The listing builds one solid part. Answer for the finished solid, in the listing's coordinates (mm). Coordinates: 2 decimals unless noted, no trailing zeros. Order: outer loops, then holes, each group sorted by start corner. A loop starts at its lowest first (then second) coordinate and runs counter-clockwise, first axis right, second up. Notation, with made-up numbers: (48, -15) -> (62, -15) arc R22 ccw to (62, 5) -> close; hole circle Ø6 at (39.5, -25). An arc over 180 degrees is marked (long way). Return JSON: item names as keys, results as strings.
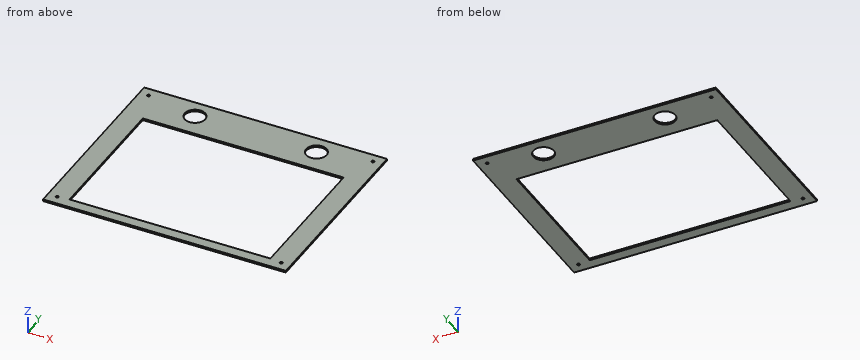
```python
from build123d import *

# Parameters (mm, degrees)
SKETCH_1_W          = 260
SKETCH_1_H          = 210
EXTRUDE_1_DEPTH     = 2
SKETCH_2_R          = 11
CUT_EXTRUDE_1_DEPTH = 2
SKETCH_3_R          = 1.5
CUT_EXTRUDE_2_DEPTH = 2
SKETCH_4_R          = 1.5
CUT_EXTRUDE_3_DEPTH = 10


with BuildPart() as part:
    # 草图1 → 凸台-拉伸1 (new body)
    with BuildSketch(Plane.XY):
        with Locations((130, 105)):
            Rectangle(SKETCH_1_W, SKETCH_1_H)
    extrude(amount=EXTRUDE_1_DEPTH)

    # 草图2 → 切除-拉伸1 (cut)
    with BuildSketch(Plane.XY.offset(2)):
        with Locations((65, 189.471035353)):
            Circle(SKETCH_2_R)
        with Locations((195, 189.471035353)):
            Circle(SKETCH_2_R)
        Polygon((130, 11.510265982), (22.5, 11.510265982), (22.5, 163.510265982), (237.5, 163.510265982), (237.5, 11.510265982), align=None)
    extrude(amount=-CUT_EXTRUDE_1_DEPTH, mode=Mode.SUBTRACT)

    # 草图3 → 切除-拉伸2 (cut)
    with BuildSketch(Plane.XY.offset(2)):
        with Locations((250, 230)):
            Circle(SKETCH_3_R)
        with Locations((10, 10)):
            Circle(SKETCH_3_R)
        with Locations((250, 10)):
            Circle(SKETCH_3_R)
        with Locations((10, 230)):
            Circle(SKETCH_3_R)
    extrude(amount=-CUT_EXTRUDE_2_DEPTH, mode=Mode.SUBTRACT)

    # 草图4 → 切除-拉伸3 (cut)
    with BuildSketch(Plane.XY.offset(2)):
        with Locations((10, 200)):
            Circle(SKETCH_4_R)
        with Locations((250, 200)):
            Circle(SKETCH_4_R)
    extrude(amount=-CUT_EXTRUDE_3_DEPTH, mode=Mode.SUBTRACT)


solid = part.part
```
Item 1: The part is cut by section A-A on x = 154. Determine the outline of the cut face in (y, z).
Answer list:
{"outline": "(0, 0) -> (11.51, 0) -> (11.51, 2) -> (0, 2) -> close; (163.51, 0) -> (210, 0) -> (210, 2) -> (163.51, 2) -> close"}
Item 2: The part is cut by section C-C on x = 195. Determine the outline of the cut face in (y, z), plus the area to 3 significant figures.
Answer list:
{"outline": "(0, 0) -> (11.51, 0) -> (11.51, 2) -> (0, 2) -> close; (163.51, 0) -> (178.47, 0) -> (178.47, 2) -> (163.51, 2) -> close; (200.47, 0) -> (210, 0) -> (210, 2) -> (200.47, 2) -> close", "area": "72.0 mm2"}
Item 3: A flat-ended cylindrical pin translates along its axis: pin 1 (1.8 mm diameter, centred on x = 10, y = 200, fed in from +Z). Find the tip coordinate at first contact, or state that the pin passes through.
Answer list:
{"pin 1": "through"}
Item 4: Find the intervals of material crossed by probe 1 along Y at (x, z) = (250, 0.45); probe 2 along X at (y, z) = (12.5, 1.4); probe 3 along Y at (x, z) = (145, 1.9), in increasing order.
Answer list:
{"probe 1": "0 to 8.5, 11.5 to 198.5, 201.5 to 210", "probe 2": "0 to 22.5, 237.5 to 260", "probe 3": "0 to 11.51, 163.51 to 210"}
Item 5: The part is cut by section D-D on z = 0.75. Determine the outline of the cut face in (x, y), plus the area to 3 significant figures.
Answer list:
{"outline": "(0, 0) -> (260, 0) -> (260, 210) -> (0, 210) -> close; hole circle Ø3 at (10, 10); hole circle Ø3 at (10, 200); hole (22.5, 11.51) -> (237.5, 11.51) -> (237.5, 163.51) -> (22.5, 163.51) -> close; hole circle Ø22 at (65, 189.47); hole circle Ø22 at (195, 189.47); hole circle Ø3 at (250, 10); hole circle Ø3 at (250, 200)", "area": "21,100 mm2"}
Item 6: The part is cut by section B-B on y = 82. Determine the outline of the cut face in (x, z).
Answer list:
{"outline": "(0, 0) -> (22.5, 0) -> (22.5, 2) -> (0, 2) -> close; (237.5, 0) -> (260, 0) -> (260, 2) -> (237.5, 2) -> close"}
